Autodesk Inventor part; units mm, degrees
ref_plane "YZ Plane" through (0, 0, 0) normal (1, 0, 0) x (0, 1, 0)
ref_plane "XZ Plane" through (0, 0, 0) normal (0, 1, 0) x (-1, 0, 0)
ref_plane "XY Plane" through (0, 0, 0) normal (0, 0, 1) x (1, 0, 0)
sketch "Sketch1" plane through (0, 0, 0) normal (0, 1, 0) x (-1, 0, 0)
  line L0 (0, 0) -> (-48, 0) construction
  line L1 (-24, 0) -> (-24, 34) construction
  line L2 (-24, 34) -> (-37.25, 34) construction
  line L3 (-24, 34) -> (-10.75, 34) construction
  circle A0 centre (-48, 0) radius 1.6
  circle A1 centre (-37.25, 34) radius 1.6
  circle A2 centre (0, 0) radius 1.6
  circle A3 centre (-10.75, 34) radius 1.6
  arc A4 (-51.8139, 1.2059) -> (-48, -4) centre (-48, 0) ccw
  arc A5 (-33.25, 34) -> (-41.0639, 35.2059) centre (-37.25, 34) ccw
  arc A6 (0, -4) -> (3.8139, 1.2059) centre (0, 0) ccw
  arc A7 (-6.9361, 35.2059) -> (-14.75, 34) centre (-10.75, 34) ccw
  arc A8 (-33.25, 34) -> (-14.75, 34) centre (-24, 34) ccw
  line L4 (0, -4) -> (-48, -4)
  line L5 (-51.8139, 1.2059) -> (-41.0639, 35.2059)
  line L6 (3.8139, 1.2059) -> (-6.9361, 35.2059)
  dimension "d0" = 48
  dimension "d1" = 34
  dimension "d2" = 13.25
  dimension "d3" = 3.2
  dimension "d4" = 3.2
  dimension "d5" = 8
  dimension "d6" = 8
extrude "Extrusion1" add sketch "Sketch1" along normal blind 2
properties part number "front mount base"
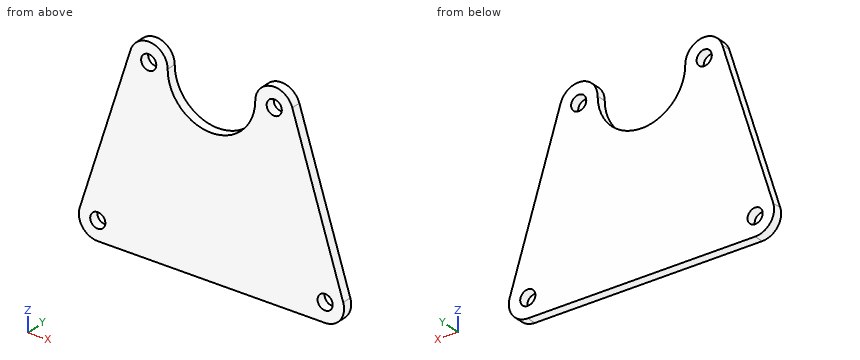
Read the model definition and answer for the solid it produces. Units are mm, in the model's axes. Give positions to 0.01 mm unless a question says otherwise; leave off trailing zeros. Write each loop counter-clockwise with the first axis right and the second up, starting at its lowest first coordinate (ties: lowest second). Pieces come first, ordered by that corner, then holes. Notation, with made-up numbers: (46.5, 32) -> (81.5, 32) arc R24 cw to (81.5, 56) -> close; hole circle Ø4 at (31.25, 82). An arc over 180 degrees is marked (long way). Answer as a JSON object with one key per item and string values.
1) Straight lines are drawn through the part: probe 1 along Z at (x, y) = (10.75, 1.4); probe 2 along X at (y, z) = (0.65, 1); probe 3 along X at (y, z) = (1.05, 8). For each, find the intervals that lie inside material, in ascending order. Write a range as from..to.
Findings below:
{"probe 1": "z = -4..32.4, 35.6..38", "probe 2": "x = -3.87..-1.25, 1.25..46.75, 49.25..51.87", "probe 3": "x = -1.67..49.67"}
2) Section A-A on z = 0 is taken. Write down the section's boundary in (x, y), then the cut area to 3 significant figures.
Findings below:
{"outline": "(-4, 0) -> (-1.6, 0) -> (-1.6, 2) -> (-4, 2) -> close; (1.6, 0) -> (46.4, 0) -> (46.4, 2) -> (1.6, 2) -> close; (49.6, 0) -> (52, 0) -> (52, 2) -> (49.6, 2) -> close", "area": "99.2 mm^2"}
3) Section C-C on x = 37.25 is taken. Write down the section's boundary in (y, z).
Findings below:
{"outline": "(0, -4) -> (2, -4) -> (2, 32.4) -> (0, 32.4) -> close; (0, 35.6) -> (2, 35.6) -> (2, 38) -> (0, 38) -> close"}
4) Section D-D on z = 29 is taken. Write down the section's boundary in (x, y), then the cut area to 3 significant figures.
Findings below:
{"outline": "(4.97, 0) -> (16.22, 0) -> (16.22, 2) -> (4.97, 2) -> close; (31.78, 0) -> (43.03, 0) -> (43.03, 2) -> (31.78, 2) -> close", "area": "45.0 mm^2"}
5) Section B-B on y = 1.35 is taken. Write down the section's boundary in (x, z), then the cut area to 3 significant figures.
Findings below:
{"outline": "(-3.81, 1.21) arc R4 ccw to (0, -4) -> (48, -4) arc R4 ccw to (51.81, 1.21) -> (41.06, 35.21) arc R4 ccw to (33.25, 34) arc R9.25 cw to (14.75, 34) arc R4 ccw to (6.94, 35.21) -> close; hole circle Ø3.2 at (0, 0); hole circle Ø3.2 at (10.75, 34); hole circle Ø3.2 at (37.25, 34); hole circle Ø3.2 at (48, 0)", "area": "1,650 mm^2"}
